Work out the finished part from the listing and answer in its coordinate system (mm). Face numbers are marked on the shaded views. A direction names the side the tool comes from. Round coordinates to 2 decimals unless told otherwise and drop trailing zeros. Order: outer loops, then holes, each group sorted by start corner. A loop starts at its lowest first (then second) coordinate and runs counter-clockwise, first axis right, second up.
from build123d import *

# Parameters (mm, degrees)
F0_W     = 30
F0_H     = 21.2
F1_DEPTH = 1.2
F2_W     = 30
F2_H     = 1.2
F3_DEPTH = 30
F4_W     = 1.2
F4_H     = 31.2
F5_DEPTH = 18.4
F6_W     = 6
F6_H     = 31.2
F7_DEPTH = 28.8
F8_W     = 28.8
F8_H     = 1.2
F9_DEPTH = 12.4


with BuildPart() as f1:
    # F0 (on Top) → F1 (new body)
    with BuildSketch(Plane.XY):
        with Locations((15, -10.6)):
            Rectangle(F0_W, F0_H)
    extrude(amount=F1_DEPTH)

    # F2 (on face) → F3 (join)
    with BuildSketch(Plane.XY.offset(1.2)):
        with Locations((15, -0.6)):
            Rectangle(F2_W, F2_H)
    extrude(amount=F3_DEPTH)

    # F4 (on face) → F5 (join)
    with BuildSketch(Plane(origin=(0, 0, 0), x_dir=(-1, 0, 0), z_dir=(0, 1, 0))):
        with Locations((-0.6, 15.6)):
            Rectangle(F4_W, F4_H)
    extrude(amount=F5_DEPTH)

    # F6 (on face) → F7 (join)
    with BuildSketch(Plane.YZ.offset(1.2)):
        with Locations((15.4, 15.6)):
            Rectangle(F6_W, F6_H)
    extrude(amount=F7_DEPTH)

    # F8 (on face) → F9 (join, through all)
    with BuildSketch(Plane.XZ.offset(-12.4)):
        with Locations((15.6, 30.6)):
            Rectangle(F8_W, F8_H)
    extrude(amount=F9_DEPTH)


solid = f1.part
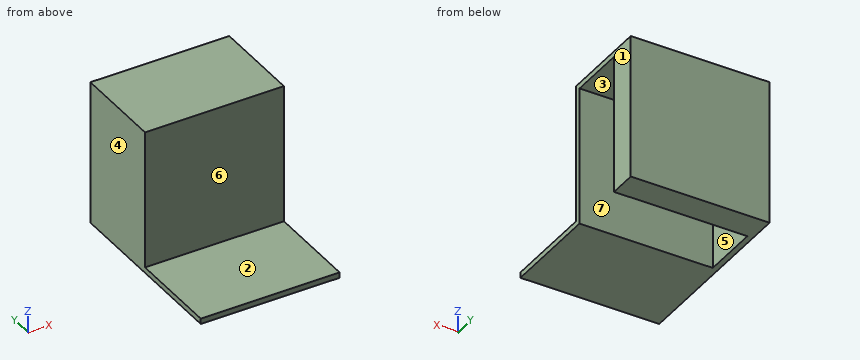
Item 1: Find the intervals of material crossed by line 1 along Y through (x, z) = (23.25, 17.5); line 2 along X through (y, z) = (7.5, 13), in increasing order.
Item 2: For a pull along Y with two mould halves and no side action, classify the marked faces 4, 5, 6 and 7 as released by +Y, released by -Y, zero draft, split by the parting line, or undercut.
Item 3: Given pin 1 (4 mm diameter, centred on x = 3.5, y = 2.5, fed in from -Z); pin 2 (8.5 mm diameter, centred on x = 18.5, z = 12, fed in from -Y); pin 3 (10 mm diameter, centred on y = 6, z = 13.5, fed in from +X), each flat-ended and moving along its own axis, determine where each tip first touches the part or whether it passes through.
Item 4: A tool of negligible diameter and unlimited length cuts with its end or side. For the marked faces 1, 2 and 3, from which of +Z, -Z, +X, -X, +Y, -Y can it reach the whole face along a straight path? Write none if from no direction.
Item 5: Find section D-D (y = -9.5). Write down the section's boundary in (x, z), plus the area to 3 significant figures.
Item 6: Find section C-C (y = 3). Write down the section's boundary in (x, z), plus the area to 3 significant figures.
Item 7: Find section B-B (z = 10). Write down the section's boundary in (x, y), plus the area to 3 significant figures.
Item 8: Find section A-A (x = 9.25). Write down the section's boundary in (y, z), plus the area to 3 significant figures.
Model answer:
1. line 1: y = -1.2 to 0, 12.4 to 18.4
1. line 2: x = 0 to 1.2
2. face 4: zero draft
2. face 5: undercut
2. face 6: released by -Y
2. face 7: undercut
3. pin 1: stops at z = 30
3. pin 2: stops at y = -1.2
3. pin 3: stops at x = 1.2
4. face 1: +Z, -Z, +X, +Y, -Y
4. face 2: +Z, +X, -X, -Y
4. face 3: -Z, +X
5. outline: (0, 0) - (30, 0) - (30, 1.2) - (0, 1.2) - close
5. area: 36.0 mm2
6. outline: (0, 0) - (1.2, 0) - (1.2, 30) - (30, 30) - (30, 31.2) - (0, 31.2) - close
6. area: 72.0 mm2
7. outline: (0, -1.2) - (30, -1.2) - (30, 0) - (1.2, 0) - (1.2, 12.4) - (30, 12.4) - (30, 18.4) - (0, 18.4) - close
7. area: 231 mm2
8. outline: (-21.2, 0) - (0, 0) - (0, 30) - (12.4, 30) - (12.4, 0) - (18.4, 0) - (18.4, 31.2) - (-1.2, 31.2) - (-1.2, 1.2) - (-21.2, 1.2) - close
8. area: 264 mm2
